CAD build for the part. Positions are in the model's coordinates, mm. Face numbers are marked on the shaded views. Round coordinates to 2 decimals unless told otherwise and drop trailing zeros. Write each loop counter-clockwise with the first axis right and the second up, starting at its lowest first coordinate (ties: lowest second). Pieces come first, ordered by that corner, then holes. Notation, with made-up numbers: (8, 46) - (62, 46) arc R36 ccw to (62, 80) - close; hole circle Ø8 at (-39.5, -22.5). An arc over 180 degrees is marked (long way). Use one line per item in the form item = value. Start each with the question number.
Item 1: Drill centre lines: L1, parallel to Z at x = 0.9, y = -0.35; L2, parallel to Z at x = -0.15, y = 0.75; L3, parallel to Y at x = -1.95, z = 2. Where is each one in solid material? Low to high.
Item 2: Band-saw the part on A-A, the plane y = -0.5. List the corners of the cut face in (x, z) (3 decimals), and give its area (3 significant figures).
Item 3: Pin check, flat tips, straight feed: pin 1 (2 mm diameter, centred on x = 1, y = -1, fed in from -Z); pin 2 (1.1 mm diameter, centred on x = -2.5, z = 1.5, fed in from -Y); pin 3 (1.5 mm diameter, centred on y = -0.5, z = 2, fed in from +X). Stop position of each tip, or through.
Item 4: Pull direction Z, two halves, no side cores. Call the marked faces 1, 2 and 3: +Z half, -Z half, draft (parallel to the pull), parting line (faces both ways), or undercut.
from build123d import *

# Parameters (mm, degrees)
EXTRUDE_1_DEPTH    = 2.4
SKETCH_2_R         = 2.75
EXTRUDE_2_DEPTH    = 1.5
FILLET_1_R         = 0.5
HOLE_WIZARD_M3_1_D = 2.5


with BuildPart() as part:
    # 草图1 → 凸台-拉伸1 (new body)
    with BuildSketch(Plane(origin=(0, 0, 0), x_dir=(1, 0, 0), z_dir=(0, 1, 0))):
        Polygon((0, 3.175426481), (-2.75, 1.58771324), (-2.75, -1.58771324), (0, -3.175426481), (2.75, -1.58771324), (2.75, 1.58771324), align=None)
    extrude(amount=EXTRUDE_1_DEPTH)

    # 草图2 → 凸台-拉伸2 (add)
    with BuildSketch(Plane.XZ):
        with Locations(Location((0, 0, 0), (0, 0, 120))):
            Circle(SKETCH_2_R)
    extrude(amount=EXTRUDE_2_DEPTH)

    # 圆角1
    fillet_1_edges = [part.edges().sort_by_distance(p)[0] for p in [
        (1.375, -1.5, -2.38156986),
    ]]
    fillet(fillet_1_edges, radius=FILLET_1_R)

    # M3 螺纹孔1 (through all)
    with Locations(Plane(origin=(0, -1.5, 0), x_dir=(-1, 0, 0), z_dir=(0, -1, 0))):
        with Locations((0, 0)):
            Hole(HOLE_WIZARD_M3_1_D / 2)

    # 草图7 → 切除-旋转2 (revolve, cut)
    with BuildSketch(Plane(origin=(0, 0, 0), x_dir=(0, 0, -1), z_dir=(1, 0, 0)), mode=Mode.PRIVATE) as cut_revolve_2_sk:
        Polygon((-3.271284624, 2.165513719), (-2.967407764, 2.4), (-3.334569784, 2.4), align=None)
        Polygon((-3.334569784, 0), (-3.271284624, 0.234486281), (-2.967407764, 0), align=None)
    revolve(cut_revolve_2_sk.sketch.rotate(Axis((0, 0, 0), (0, 1, 0)), 180), axis=Axis((0, 0, 0), (0, 1, 0)), mode=Mode.SUBTRACT)


solid = part.part
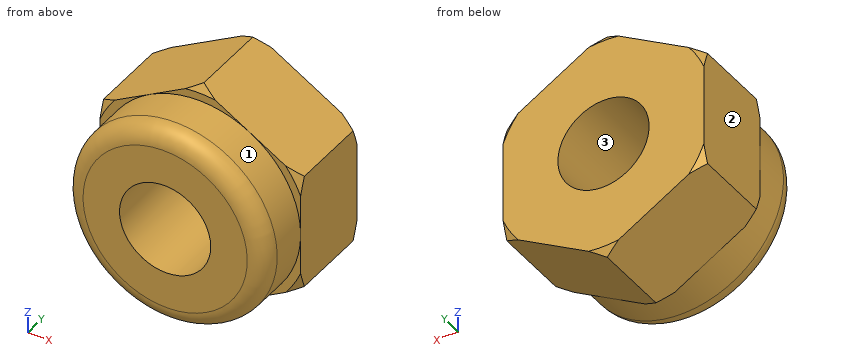
Determined:
q1.L1 = -2.6 to -0.87, 0.87 to 2.6
q1.L2 = -3.09 to -1.24, 1.24 to 3.09
q1.L3 = 0 to 2.4
q2.outline = circle Ø5.5 at (0, 0); hole circle Ø2.5 at (0, 0)
q2.area = 18.8 mm²
q3.pin_1 = -2.75
q3.pin_2 = -1.49
q3.pin_3 = 2.71
q4.face_1 = parting line
q4.face_2 = draft
q4.face_3 = undercut
